from build123d import *

# Parameters (mm, degrees)
SKETCH1_R           = 3.7465
SKETCH1_R_2         = 1.25
BOSS_EXTRUDE1_DEPTH = 3


with BuildPart() as part:
    # Sketch1 → Boss-Extrude1 (new body)
    with BuildSketch(Plane.XY):
        with BuildLine():
            Line((-5, -42), (-5, -39))
            ThreePointArc((-5, -39), (-3.64832327, -37.196831118), (-1.538417978, -37.988505079))
            ThreePointArc((-1.538417978, -37.988505079), (-0.839409352, -39.527103714), (-0.6, -41.2))
            ThreePointArc((-0.6, -41.2), (0, -43), (0.6, -41.2))
            ThreePointArc((0.6, -41.2), (0.210597624, -38.870174368), (-0.915279992, -36.793609589))
            ThreePointArc((-0.915279992, -36.793609589), (-1.38227286, -35.62821691), (-1.15567211, -34.393358808))
            ThreePointArc((-1.15567211, -34.393358808), (1.906967722, -23.36077989), (0.613240327, -11.984320436))
            ThreePointArc((0.613240327, -11.984320436), (-5.611566101, 10.607088474), (9.562398428, -7.249864571))
            ThreePointArc((9.562398428, -7.249864571), (11.572717875, -26.830951895), (4, -45))
            ThreePointArc((4, -45), (-1.58113883, -46.74341649), (-5, -42))
        make_face()
        Circle(SKETCH1_R, mode=Mode.SUBTRACT)
        with Locations((0, 8.509)):
            Circle(SKETCH1_R_2, mode=Mode.SUBTRACT)
        with Locations((-7.62, 0)):
            Circle(SKETCH1_R_2, mode=Mode.SUBTRACT)
        with Locations((0, -8.509)):
            Circle(SKETCH1_R_2, mode=Mode.SUBTRACT)
        with Locations((7.62, 0)):
            Circle(SKETCH1_R_2, mode=Mode.SUBTRACT)
    extrude(amount=BOSS_EXTRUDE1_DEPTH)


solid = part.part
Can you work these out from the model? Positions are in its coordinate system, mm. A direction names the side the tool comes from. Give positions to 0.01 mm unless a question says otherwise; leave off trailing zeros. Order: outer loops, then holes, each group sorted by start corner. A loop starts at its lowest first (then second) coordinate and runs counter-clockwise, first axis right, second up. Notation, with made-up numbers: (-20.75, 56) - (-1.75, 56) arc R21 ccw to (-1.75, 90) - close; hole circle Ø4 at (55, 44.5). An arc over 180 degrees is marked (long way). Write each question's results on one line, items separated by ' | '.
1) On a 3-axis mill with a long thin cutter (end or side, diameter ignored), from which of +Z, -Z, +X, -X, +Y, -Y can I reach the whole of each face in a straight line? I mean faces 4 (the face through (-0.846, -39.504, 1.479)), 5 (the face through (3, -11, 0)). Say none if no direction works.
Final values:
face 4: +Z, -Z | face 5: -Z, +X, -X, +Y, -Y
2) If we mould it in two halves opening along X, with no side actions, what happens to faces 1 (the face through (-1.5, -46.77, 1.48)), 2 (the face through (6.37, 0.05, 1.48)), 3 (the face through (-5, -41, 1))? For each: pulls with the +X half, pulls with the -X half, needs draft (parallel to the pull), parting line crosses it, or undercut.
Final values:
face 1: parting line crosses it | face 2: undercut | face 3: pulls with the -X half
3) I'm going to push flat-ended pins straight in: pin 1 Ø2 at (x, y) = (0, -8.509) entering from -Z; pin 2 Ø1.5 at (x, z) = (8, 2) entering from +Y; pin 3 Ø1.5 at (y, z) = (-31, 2) entering from -X; pin 4 Ø0.9 at (y, z) = (-40.5, 1) entering from -X. Where does each tip first touch, or does it pass through?
Final values:
pin 1: passes through | pin 2: stops at y = 9.56 | pin 3: stops at x = 0.01 | pin 4: stops at x = -5
4) Suppose I cut it at A-A, the plane y = 0. Write out the boundary of the cut face in (x, z), then the cut area to 3 significant figures.
Final values:
outline: (-12, 0) - (-8.87, 0) - (-8.87, 3) - (-12, 3) - close; (-6.37, 0) - (-3.75, 0) - (-3.75, 3) - (-6.37, 3) - close; (3.75, 0) - (6.37, 0) - (6.37, 3) - (3.75, 3) - close; (8.87, 0) - (12, 0) - (12, 3) - (8.87, 3) - close | area: 34.5 mm^2
5) Suppose I cut it at B-B, the plane z = 0.45. Write out the boundary of the cut face in (x, y).
Final values:
outline: (-5, -42) arc R5 ccw to (4, -45) arc R40 ccw to (9.56, -7.25) arc R12 ccw (long way) to (0.61, -11.98) arc R30 cw to (-1.16, -34.39) arc R2.26 ccw to (-0.92, -36.79) arc R7.16 cw to (0.6, -41.2) arc R1 cw (long way) to (-0.6, -41.2) arc R5.96 ccw to (-1.54, -37.99) arc R1.88 ccw to (-5, -39) - close; hole circle Ø2.5 at (-7.62, 0); hole circle Ø7.49 at (0, 0); hole circle Ø2.5 at (0, -8.51); hole circle Ø2.5 at (0, 8.51); hole circle Ø2.5 at (7.62, 0)
6) Suppose I cut it at D-D, the plane x = 0. Write out the boundary of the cut face in (y, z).
Final values:
outline: (-47, 0) - (-43, 0) - (-43, 3) - (-47, 3) - close; (-38.33, 0) - (-31.77, 0) - (-31.77, 3) - (-38.33, 3) - close; (-12, 0) - (-9.76, 0) - (-9.76, 3) - (-12, 3) - close; (-7.26, 0) - (-3.75, 0) - (-3.75, 3) - (-7.26, 3) - close; (3.75, 0) - (7.26, 0) - (7.26, 3) - (3.75, 3) - close; (9.76, 0) - (12, 0) - (12, 3) - (9.76, 3) - close
7) Suppose I cut it at C-C, the plane x = -7.62. Write out the boundary of the cut face in (y, z), then the cut area to 3 significant figures.
Final values:
outline: (-9.27, 0) - (-1.25, 0) - (-1.25, 3) - (-9.27, 3) - close; (1.25, 0) - (9.27, 0) - (9.27, 3) - (1.25, 3) - close | area: 48.1 mm^2
8) Please list where these lines run through material, in increasing order: line 1 along Y through (x, z) = (-0.25, 1.5); line 2 along Y through (x, z) = (-2, 2.3); line 3 along Y through (x, z) = (7.62, 1.1). Write a range as [from, to].
Final values:
line 1: y = [-46.99, -42.97], [-37.82, -32.4], [-12, -9.73], [-7.28, -3.74], [3.74, 7.28], [9.73, 12] | line 2: y = [-46.58, -37.49], [-11.83, -3.17], [3.17, 11.83] | line 3: y = [-39.2, -1.25], [1.25, 9.27]
